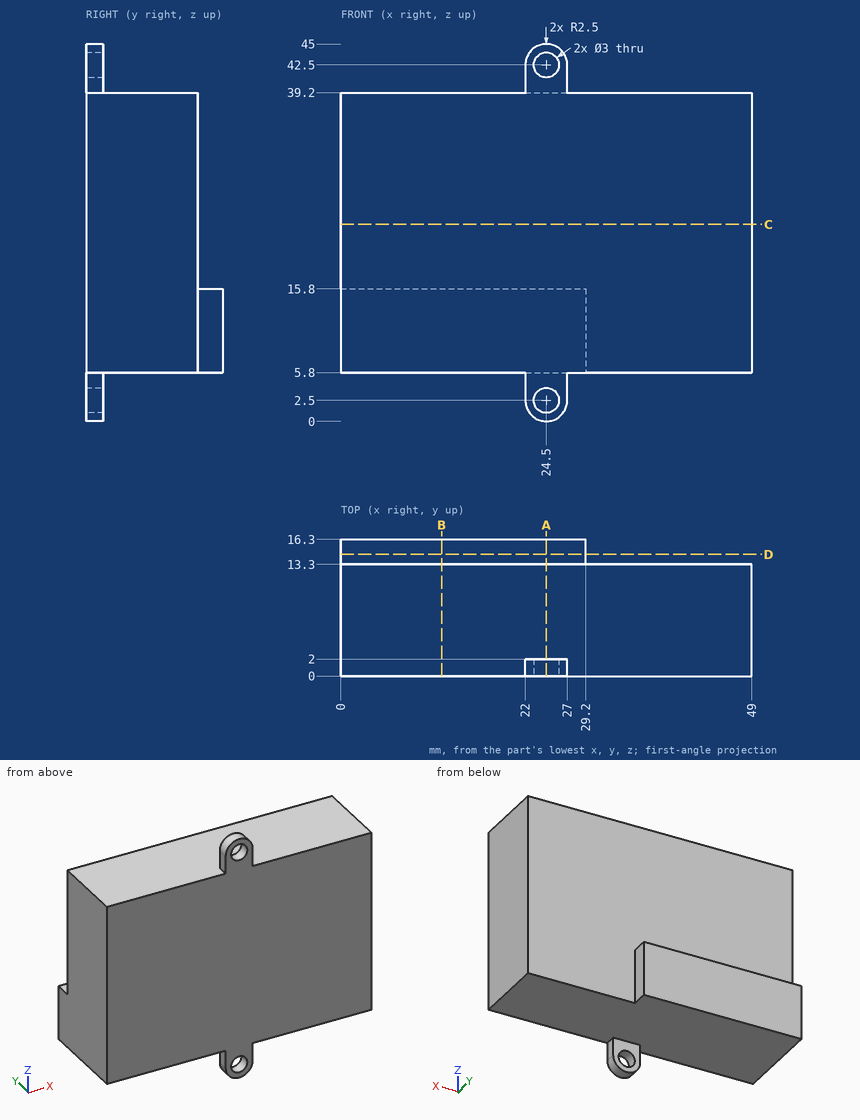
Check sheet for the drawn part. Datum: minimum x, y, z corner. Units: mm. Round coordinates to 2 decimals unless told otherwise and drop trailing zeros. Order: outer loops, then holes, each group sorted by start corner. A loop starts at its lowest first (then second) coordinate and runs counter-clockwise, first axis right, second up. Notation, with made-up numbers: (-35.75, 49) - (-0.75, 49) arc R20 cw to (-0.75, 60) - close; hole circle Ø1 at (17, 60.25). An arc over 180 degrees is marked (long way). Use a Markdown table: item, result. Add a question column.
(1) Sectioned sample at D-D, the plane y = 14.5. Enter the section's corners in (x, z).
(2) Sectioned sample at C-C, the plane z = 23.5. Enter the section's corners in (x, y).
(3) Depth check by flat-ended pin: pin 1 (1.5 mm diameter, centred on x = 25, y = 9, fed in from +Z); pin 2 (1.5 mm diameter, centred on x = 20, z = 20, fed in from +Y); pin 3 (1.5 mm diameter, centred on x = 29.5, y = 13.5, fed in from -Z). Enter the tip coordinate at first touch or a pass-through.
(4) Sectioned sample at A-A, the plane x = 24.5. Enter the section's corners in (y, z), and give its area (3 significant figures).
(5) Sectioned sample at B-B, the plane x = 12. Enter the section's corners in (y, z), and give its area (3 significant figures).
(6) Material ranges on line 1 along X through (y, z) = (1.55, 42.5); line 2 along Z through (x, y) = (8, 13); line 3 along Y through (x, z) = (32, 33), recorded low to high. Write a range as [from, to].
Answers below:
| question | item | result |
|---|---|---|
| 1 | outline | (0, 5.8) - (29.2, 5.8) - (29.2, 15.8) - (0, 15.8) - close |
| 2 | outline | (0, 0) - (49, 0) - (49, 13.3) - (0, 13.3) - close |
| 3 | pin 1 | z = 39.2 |
| 3 | pin 2 | y = 13.3 |
| 3 | pin 3 | z = 5.8 |
| 4 | outline | (0, 0) - (2, 0) - (2, 1) - (0, 1) - close; (0, 4) - (2, 4) - (2, 5.8) - (16.3, 5.8) - (16.3, 15.8) - (13.3, 15.8) - (13.3, 39.2) - (2, 39.2) - (2, 41) - (0, 41) - close; (0, 44) - (2, 44) - (2, 45) - (0, 45) - close |
| 4 | area | 485 mm² |
| 5 | outline | (0, 5.8) - (16.3, 5.8) - (16.3, 15.8) - (13.3, 15.8) - (13.3, 39.2) - (0, 39.2) - close |
| 5 | area | 474 mm² |
| 6 | line 1 | [22, 23], [26, 27] |
| 6 | line 2 | [5.8, 39.2] |
| 6 | line 3 | [0, 13.3] |
